Source: CAD feature listing. Evaluate the final solid. Frame: model axes, mm. Face numbers are marked on the shaded views. A direction names the side the tool comes from. Round coordinates to 2 decimals unless told otherwise and drop trailing zeros. Write each loop counter-clockwise with the first axis right and the second up, starting at its lowest first coordinate (ties: lowest second). Pieces come first, ordered by that corner, then holes. Notation, with made-up numbers: (-16, 10) -> (23, 10) arc R30 ccw to (23, 37) -> close; hole circle Ø11 at (41.5, 6). An arc over 180 degrees is marked (long way). Put each result on its own line as item: value.
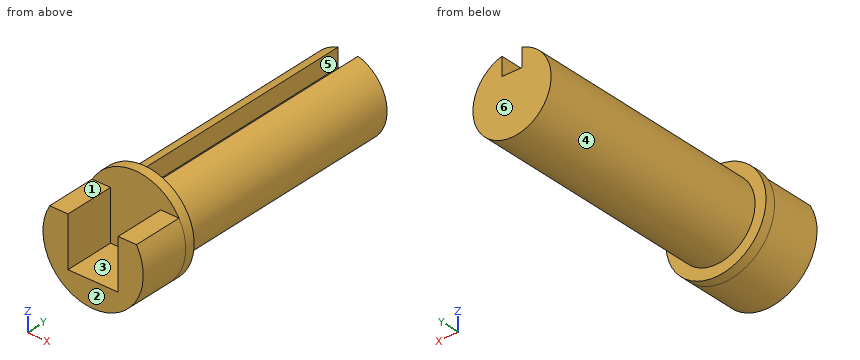
```python
from build123d import *

# Parameters (mm, degrees)
F1_DEPTH = 31.75
F2_R     = 31.75
F3_DEPTH = 6.35
F5_DEPTH = 152.4


with BuildPart() as f1:
    # F0 (on Front) → F1 (new body)
    with BuildSketch(Plane.XZ):
        with BuildLine():
            Line((-15.875, 15.875), (-27.496307, 15.875))
            ThreePointArc((-27.496307, 15.875), (0, -31.75), (27.496307, 15.875))
            Line((27.496307, 15.875), (15.875, 15.875))
            Line((15.875, 15.875), (15.875, -15.875))
            Line((15.875, -15.875), (-15.875, -15.875))
            Line((-15.875, -15.875), (-15.875, 15.875))
        make_face()
    extrude(amount=F1_DEPTH)

    # F2 (on face) → F3 (join)
    with BuildSketch(Plane(origin=(0, 0, 0), x_dir=(-1, 0, 0), z_dir=(0, 1, 0))):
        Circle(F2_R)
    extrude(amount=F3_DEPTH)

    # F4 (on face) → F5 (join)
    with BuildSketch(Plane(origin=(0, 6.35, 0), x_dir=(-1, 0, 0), z_dir=(0, 1, 0))):
        with BuildLine():
            Line((-6.35, 12.3825), (-6.35, 23.937058))
            ThreePointArc((-6.35, 23.937058), (0, -24.765), (6.35, 23.937058))
            Line((6.35, 23.937058), (6.35, 12.3825))
            Line((6.35, 12.3825), (0, 12.3825))
            Line((0, 12.3825), (-6.35, 12.3825))
        make_face()
    extrude(amount=F5_DEPTH)


solid = f1.part
```
Q1. Pin query (flat end, axial travel): pin 1 (5 mm diameter, centred on y = 41.5, z = -1, fed in from +X) (3 decimals); pin 2 (8 mm diameter, centred on y = 38, z = -14, fed in from +X); pin 3 (1 mm diameter, centred on y = 137.5, z = 22.5, fed in from +X); pin 4 (6 mm diameter, centred on x = -20, z = 18, fed in from -Y). Return the tip coordinate at first contact, or that it passes through.
Ans:
pin 1: stops at x = 24.765
pin 2: stops at x = 22.66
pin 3: stops at x = 11.37
pin 4: stops at y = -31.75
Q2. Draft query along X for the marked faces 4, 5 and 6. Return one class per face: +X half, -X half, draft (parallel to the pull), parting line (faces both ways), or undercut.
Ans:
face 4: parting line
face 5: undercut
face 6: draft
Q3. Material intervals for line 1 (Y direction, x = 6, z = 1.5); line 2 (X direction, y = 60.5, z = 14); line 3 (Y direction, x = 18, z = 21), sorted ascending. Write a range as [from, to].
Ans:
line 1: y = [0, 158.75]
line 2: x = [-20.43, -6.35], [6.35, 20.43]
line 3: y = [0, 6.35]
Q4. Cut plane A-A on z = 0. Output: boundary loops of the cut face in (x, y) (3 decimals).
Ans:
outline: (-31.75, -31.75) -> (-15.875, -31.75) -> (-15.875, 0) -> (15.875, 0) -> (15.875, -31.75) -> (31.75, -31.75) -> (31.75, 6.35) -> (24.765, 6.35) -> (24.765, 158.75) -> (-24.765, 158.75) -> (-24.765, 6.35) -> (-31.75, 6.35) -> close
Q5. Reachability of the marked faces 1, 2 and 3 from +Z, -Z, +X, -X, +Y, -Y: full face, straight path, thin tool, end or side. Return the list, or none.
Ans:
face 1: +Z, +X, -X, -Y
face 2: +Z, -Z, +X, -X, -Y
face 3: +Z, -Y
